Part model, mm, in its own coordinate system. A direction names the side the tool comes from. Coordinates: 2 decimals unless noted, no trailing zeros. Write each loop counter-clockwise with the first axis right and the second up, starting at its lowest first coordinate (ties: lowest second). Pieces come first, ordered by that corner, then holes. Notation, with made-up numbers: (82.5, -37) -> (93.5, -37) arc R23 ccw to (93.5, -4) -> close; hole circle Ø1 at (21.5, 15). An arc over 180 degrees is marked (long way). Write item = value, one per line. Start each with the question number.
Q1. Tool access for faces 1 (the cylindrical face through (79.964, 10.14, 80.742)), 2 (the cylindrical face through (46.1, 71.4, -6.1)), 3 (the flat face through (-1, 10, -95)): list every direction of +Z, -Z, +X, -X, +Y, -Y with a clear straight run to the whole face (end or side of a thin tool).
Q2. Probe line 1 (X direction, y = 63, z = 0); line 2 (Y direction, x = 5.5, z = 3); line 3 (X direction, y = 83, z = 0). List the from-to ranges inside material, lowest first.
Q3. Pull direction Y, two halves, no side cores. Call faces 4 (the flat face through (74, 82.3, -20)), 5 (the flat face through (2, -10, 2)), 6 (the cylindrical face through (-80.742, 10.14, -79.964)): released by +Y, released by -Y, zero draft, split by the parting line, or undercut.
Q4. Band-saw the part on D-D, the plane x = -80. List the corners of the cut face in (y, z).
Q5. Band-saw the part on C-C, the plane y = 8.5. List the corners of the cut face in (x, z), plus the area to 3 significant figures.
Q6. Pin check, flat tips, straight feed: P1, Ø1.5, axis at y = 61.5, z = -36.5, coming from the -X side; P2, Ø10, axis at x = 67, y = 4, coming from the +Z side; P3, Ø10, axis at x = 84.5, y = 0.5, coming from the +Z side. Stop position of each tip, or through.
Q7. Band-saw the part on B-B, the plane x = 0. List the corners of the cut face in (y, z).
Q8. Band-saw the part on A-A, the plane z = 0. List the corners of the cut face in (x, y).
from build123d import *

# Parameters (mm, degrees)
SKETCH_3_W          = 190
SKETCH_3_H          = 190
EXTRUDE_3_DEPTH     = 20
FILLET_2_R          = 50
SKETCH_4_R          = 75
EXTRUDE_4_DEPTH     = 42.3
SKETCH_5_R          = 75
EXTRUDE_5_DEPTH     = 20
SKETCH_14_R         = 90
EXTRUDE_7_DEPTH     = 10
SKETCH_15_R         = 46.5
CUT_EXTRUDE_9_DEPTH = 42.3
SKETCH_12_R         = 54
EXTRUDE_6_DEPTH     = 10
SKETCH_13_R         = 46.5
CUT_EXTRUDE_7_DEPTH = 41.3
SKETCH_18_R         = 125
EXTRUDE_8_DEPTH     = 10


with BuildPart() as part:
    # 草图3 → 凸台-拉伸3 (new body)
    with BuildSketch(Plane(origin=(0, 0, 0), x_dir=(1, 0, 0), z_dir=(0, 1, 0))):
        Rectangle(SKETCH_3_W, SKETCH_3_H)
    extrude(amount=EXTRUDE_3_DEPTH)

    # 圆角2
    fillet_2_edges = [part.edges().sort_by_distance(p)[0] for p in [
        (95, 10, 95),
        (-95, 10, 95),
        (-95, 10, -95),
        (95, 10, -95),
    ]]
    fillet(fillet_2_edges, radius=FILLET_2_R)

    # 草图4 → 凸台-拉伸4 (add)
    with BuildSketch(Plane(origin=(0, 20, 0), x_dir=(1, 0, 0), z_dir=(0, 1, 0))):
        with Locations(Location((0, 0, 0), (0, 0, 270))):
            Circle(SKETCH_4_R)
    extrude(amount=EXTRUDE_4_DEPTH)

    # 草图5 → 凸台-拉伸5 (add)
    with BuildSketch(Plane(origin=(0, 62.3, 0), x_dir=(1, 0, 0), z_dir=(0, 1, 0))):
        with Locations(Location((0, 0, 0), (0, 0, 270))):
            Circle(SKETCH_5_R)
    extrude(amount=EXTRUDE_5_DEPTH)

    # 草图14 → 凸台-拉伸7 (add)
    with BuildSketch(Plane(origin=(0, 82.3, 0), x_dir=(1, 0, 0), z_dir=(0, 1, 0))):
        with Locations(Location((0, 0, 0), (0, 0, 270))):
            Circle(SKETCH_14_R)
    extrude(amount=EXTRUDE_7_DEPTH)

    # 草图15 → 切除-拉伸9 (cut)
    with BuildSketch(Plane(origin=(0, 92.3, 0), x_dir=(1, 0, 0), z_dir=(0, 1, 0))):
        with Locations(Location((0, 0, 0), (0, 0, 270))):
            Circle(SKETCH_15_R)
    extrude(amount=-CUT_EXTRUDE_9_DEPTH, mode=Mode.SUBTRACT)

    # 草图12 → 凸台-拉伸6 (add)
    with BuildSketch(Plane(origin=(0, 82.3, 0), x_dir=(1, 0, 0), z_dir=(0, 1, 0))):
        Circle(SKETCH_12_R)
    extrude(amount=EXTRUDE_6_DEPTH)

    # 草图13 → 切除-拉伸7 (cut)
    with BuildSketch(Plane(origin=(0, 92.3, 0), x_dir=(1, 0, 0), z_dir=(0, 1, 0))):
        with Locations(Location((0, 0, 0), (0, 0, 270))):
            Circle(SKETCH_13_R)
    extrude(amount=-CUT_EXTRUDE_7_DEPTH, mode=Mode.SUBTRACT)

    # 草图18 → 凸台-拉伸8 (add)
    with BuildSketch(Plane.XZ):
        with Locations(Location((0, 0, 0), (0, 0, 270))):
            Circle(SKETCH_18_R)
    extrude(amount=EXTRUDE_8_DEPTH)


solid = part.part
Ans:
q1.face_1 = +Z, +X, +Y
q1.face_2 = +Y
q1.face_3 = -Z, +X, -X, +Y
q2.line_1 = -75 to -46.5, 46.5 to 75
q2.line_2 = -10 to 50
q2.line_3 = -90 to -46.5, 46.5 to 90
q3.face_4 = undercut
q3.face_5 = released by -Y
q3.face_6 = zero draft
q4.outline = (-10, -96.05) -> (0, -96.05) -> (0, -80.71) -> (20, -80.71) -> (20, 80.71) -> (0, 80.71) -> (0, 96.05) -> (-10, 96.05) -> close; (82.3, -41.23) -> (92.3, -41.23) -> (92.3, 41.23) -> (82.3, 41.23) -> close
q5.outline = (-95, -45) arc R50 ccw to (-45, -95) -> (45, -95) arc R50 ccw to (95, -45) -> (95, 45) arc R50 ccw to (45, 95) -> (-45, 95) arc R50 ccw to (-95, 45) -> close
q5.area = 34,000 mm2
q6.P1 = -65.93
q6.P2 = 107.37
q6.P3 = 96.44
q7.outline = (-10, -125) -> (0, -125) -> (0, -95) -> (20, -95) -> (20, -75) -> (82.3, -75) -> (82.3, -90) -> (92.3, -90) -> (92.3, -46.5) -> (50, -46.5) -> (50, 46.5) -> (92.3, 46.5) -> (92.3, 90) -> (82.3, 90) -> (82.3, 75) -> (20, 75) -> (20, 95) -> (0, 95) -> (0, 125) -> (-10, 125) -> close
q8.outline = (-125, -10) -> (125, -10) -> (125, 0) -> (95, 0) -> (95, 20) -> (75, 20) -> (75, 82.3) -> (90, 82.3) -> (90, 92.3) -> (46.5, 92.3) -> (46.5, 50) -> (-46.5, 50) -> (-46.5, 92.3) -> (-90, 92.3) -> (-90, 82.3) -> (-75, 82.3) -> (-75, 20) -> (-95, 20) -> (-95, 0) -> (-125, 0) -> close
